CAD build for the part. Positions are in the model's coordinates, mm. A direction names the side the tool comes from. Round coordinates to 2 decimals unless told otherwise and drop trailing zeros. Order: outer loops, then holes, each group sorted by start corner. A loop starts at its lowest first (then second) coordinate and runs counter-clockwise, first axis right, second up. Notation, with made-up numbers: (67, 17.25) -> (94, 17.25) arc R10 ccw to (94, 28.25) -> close; hole circle Ø4 at (-26.5, 6). An arc over 180 degrees is marked (long way). Return JSON: item names as keys, results as strings. Group by question number.
Q1. Cut at B-B (y = 446.5). Write the cut outline in (x, z).
Q2. Cut at A-A (z = 17). Write the cut outline in (x, y).
Q3. Flat gauge pins, fed straight in: pin 1 (14.5 mm diameter, centred on y = 549.5, z = 16, fed in from +X); pin 2 (2 mm diameter, centred on x = 15.5, y = 294, fed in from +Z); pin 3 (1.2 mm diameter, centred on y = 399.5, z = 32, fed in from +X); pin 4 (2.5 mm diameter, centred on x = 11.5, z = 9.5, fed in from -Y). Where does each tip first touch, or does it go through?
Q4. Probe line 1 along Y through (x, z) = (9.25, 27); line 2 along Z through (x, y) = (16.5, 524.5); line 3 along X through (y, z) = (32.5, 32). List the from-to ranges inside material, lowest first.
Q5. Which spindle directions (+Z, -Z, +X, -X, +Y, -Y) get a long thin tool onto all of the face, cutting with end or side? Do faces 1 (the flat face through (9, 553, 18)), 2 (the flat face through (13, 18, 17)), 3 (the flat face through (4, 562, 17)). Say none if no direction does.
from build123d import *

# Parameters (mm, degrees)
F0_W     = 526
F0_H     = 31
F1_DEPTH = 18
F0_W_2   = 18
F0_H_2   = 4
F2_DEPTH = 9
F3_DEPTH = 14


with BuildPart() as f1:
    # F0 (on Right) → F1 (new body)
    with BuildSketch(Plane.YZ):
        with Locations((281, 15.5)):
            Rectangle(F0_W, F0_H)
    extrude(amount=F1_DEPTH)

    # F0 (on Right) → F2 (join)
    with BuildSketch(Plane.YZ):
        with Locations((9, 15.5)):
            Rectangle(F0_W_2, F0_H)
        with Locations((553, 15.5)):
            Rectangle(F0_W_2, F0_H)
        with Locations((9, 33)):
            Rectangle(F0_W_2, F0_H_2)
        with Locations((553, 33)):
            Rectangle(F0_W_2, F0_H_2)
    extrude(amount=F2_DEPTH)

    # F0 (on Right) → F3 (join)
    with BuildSketch(Plane.YZ):
        with Locations((281, 33)):
            Rectangle(F0_W, F0_H_2)
    extrude(amount=F3_DEPTH)


solid = f1.part
Solution:
{
 "1": {"outline": "(0, 0) -> (18, 0) -> (18, 31) -> (14, 31) -> (14, 35) -> (0, 35) -> close"},
 "2": {"outline": "(0, 0) -> (9, 0) -> (9, 18) -> (18, 18) -> (18, 544) -> (9, 544) -> (9, 562) -> (0, 562) -> close"},
 "3": {"pin 1": "stops at x = 18", "pin 2": "stops at z = 31", "pin 3": "stops at x = 14", "pin 4": "stops at y = 18"},
 "4": {"line 1": "y = 18 to 544", "line 2": "z = 0 to 31", "line 3": "x = 0 to 14"},
 "5": {"face 1": "+Z, -Z, +X, +Y", "face 2": "+Z, -Z, +X, -Y", "face 3": "+Z, -Z, +X, -X, +Y"}
}
